CAD build for the part. Positions are in the model's coordinates, mm. A direction names the side the tool comes from. Coordinates: 2 decimals unless noted, no trailing zeros. Write each question's results on one line, items separated by ' | '.
```python
from build123d import *

# Parameters (mm, degrees)
F0_W      = 630
F0_H      = 830
F1_DEPTH  = 25
F2_W      = 40
F2_H      = 40
F3_DEPTH  = 25
F4_W      = 40
F4_H      = 40
F5_DEPTH  = 25
F6_W      = 40
F6_H      = 40
F7_DEPTH  = 25
F8_W      = 40
F8_H      = 40
F9_DEPTH  = 25
F10_R     = 3
F11_DEPTH = 25


with BuildPart() as f1:
    # F0 (on Top) → F1 (new body)
    with BuildSketch(Plane.XY):
        with Locations((315, 415)):
            Rectangle(F0_W, F0_H)
    extrude(amount=F1_DEPTH)

    # F2 (on face) → F3 (cut)
    with BuildSketch(Plane.XY.offset(25)):
        with Locations((610, 20)):
            Rectangle(F2_W, F2_H)
    extrude(amount=-F3_DEPTH, mode=Mode.SUBTRACT)

    # F4 (on face) → F5 (cut)
    with BuildSketch(Plane.XY.offset(25)):
        with Locations((20, 20)):
            Rectangle(F4_W, F4_H)
    extrude(amount=-F5_DEPTH, mode=Mode.SUBTRACT)

    # F6 (on face) → F7 (cut)
    with BuildSketch(Plane(origin=(0, 0, 0), x_dir=(1, 0, 0), z_dir=(0, 0, -1))):
        with Locations((20, -810)):
            Rectangle(F6_W, F6_H)
    extrude(amount=-F7_DEPTH, mode=Mode.SUBTRACT)

    # F8 (on face) → F9 (cut)
    with BuildSketch(Plane(origin=(0, 0, 0), x_dir=(1, 0, 0), z_dir=(0, 0, -1))):
        with Locations((610, -810)):
            Rectangle(F8_W, F8_H)
    extrude(amount=-F9_DEPTH, mode=Mode.SUBTRACT)

    # F10 (on face) → F11 (cut)
    with BuildSketch(Plane(origin=(40, 0, 0), x_dir=(0, -1, 0), z_dir=(-1, 0, 0))):
        with Locations((-20, 12.5)):
            Circle(F10_R)
    extrude(amount=-F11_DEPTH, mode=Mode.SUBTRACT)


solid = f1.part
```
Q1. Which spindle directions (+Z, -Z, +X, -X, +Y, -Y) get a long thin tool onto all of the face, cutting with end or side? Do faces 1 (the flat face through (20, 790, 12)), 2 (the flat face through (630, 410, 12)), 3 (the flat face through (40, 24, 13)), 4 (the flat face through (610, 790, 12)), 5 (the flat face through (610, 40, 13)). Say none if no direction does.
Results are:
face 1: +Z, -Z, -X, +Y | face 2: +Z, -Z, +X, +Y, -Y | face 3: +Z, -Z, -X, -Y | face 4: +Z, -Z, +X, +Y | face 5: +Z, -Z, +X, -Y
Q2. Drop flat-ended pins along their axis: pin 1 (7 mm diameter, centred on y = 20, z = 12.5, fed in from -X); pin 2 (12.5 mm diameter, centred on x = 28.5, z = 11, fed in from -Y); pin 3 (12.5 mm diameter, centred on y = 809, z = 12.5, fed in from +X). Give the stop position or say it passes through.
Results are:
pin 1: x = 40 | pin 2: y = 40 | pin 3: x = 590
Q3. Wall check: L1, parallel to Z at x = 45, y = 20. Give the ranges that are in metal, low to high. Write a range as from..to.
Results are:
L1: 0..9.5, 15.5..25
Q4. Pull direction Y, two halves, no side cores. Call faces 6 (the flat face through (40, 810, 12)), 7 (the flat face through (20, 40, 13)), 8 (the flat face through (311, 830, 12)): +Y half, -Y half, draft (parallel to the pull), parting line (faces both ways), or undercut.
Results are:
face 6: draft | face 7: -Y half | face 8: +Y half
